Verification items for this drawing (mm, ordinates from the low corner). Round coordinates to 2 decimals unless told otherwise and drop trailing zeros. Order: outer loops, then holes, each group sorted by start corner. A loop starts at its lowest first (then second) coordinate and runs counter-clockwise, first axis right, second up. Notation, with made-up numbers: (-22, 69.25) -> (32, 69.25) arc R21 cw to (32, 87.25) -> close; hole circle Ø1 at (63, 27.25). An arc over 180 degrees is marked (long way). Put each result on its own line as item: value.
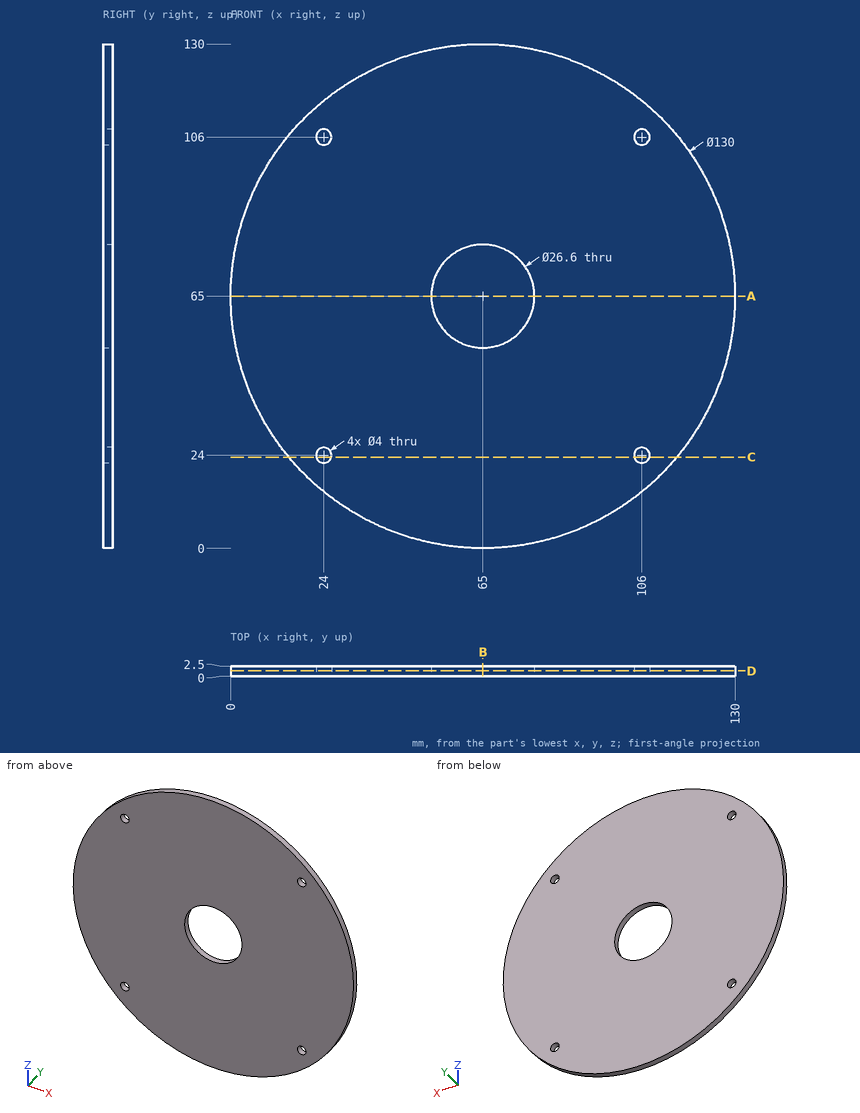
Item 1: Material ranges on L1, parallel to X at y = 1.05, z = 106; L2, parallel to X at y = 1.3, z = 59; L3, parallel to X at y = 1.1, z = 68.5, recorded low to high. Write a range as [from, to].
Check sheet entries:
L1: x = [14.56, 22], [26, 104], [108, 115.44]
L2: x = [0.28, 53.13], [76.87, 129.72]
L3: x = [0.09, 52.17], [77.83, 129.91]
Item 2: Gauge pin test, flat end, axial feed: pin 1 Ø2 at (x, z) = (69, 36.5) entering from -Y. Record the tip position at first contact, or that the pin passes through.
Check sheet entries:
pin 1: stops at y = 0
Item 3: Section check D-D on y = 1.3. Record the boundary of the cut face in (x, z).
Check sheet entries:
outline: circle Ø130 at (65, 65); hole circle Ø4 at (24, 24); hole circle Ø4 at (24, 106); hole circle Ø26.6 at (65, 65); hole circle Ø4 at (106, 24); hole circle Ø4 at (106, 106)
Item 4: Section check C-C on z = 23.5. Record the boundary of the cut face in (x, y).
Check sheet entries:
outline: (14.97, 0) -> (22.06, 0) -> (22.06, 2.5) -> (14.97, 2.5) -> close; (25.94, 0) -> (104.06, 0) -> (104.06, 2.5) -> (25.94, 2.5) -> close; (107.94, 0) -> (115.03, 0) -> (115.03, 2.5) -> (107.94, 2.5) -> close
Item 5: Section check B-B on x = 65. Record the boundary of the cut face in (y, z).
Check sheet entries:
outline: (0, 0) -> (2.5, 0) -> (2.5, 51.7) -> (0, 51.7) -> close; (0, 78.3) -> (2.5, 78.3) -> (2.5, 130) -> (0, 130) -> close
Item 6: Section check A-A on z = 65. Record the boundary of the cut face in (x, y), then the cut area to 4 significant figures.
Check sheet entries:
outline: (0, 0) -> (51.7, 0) -> (51.7, 2.5) -> (0, 2.5) -> close; (78.3, 0) -> (130, 0) -> (130, 2.5) -> (78.3, 2.5) -> close
area: 258.5 mm^2
